The model under review builds one solid part; all positions refer to its coordinate system, in mm. Face numbers are marked on the shaded views. Give positions to 0.01 mm unless a question says otherwise; leave off trailing zeros. Loops run counter-clockwise (first coordinate to the right, second up) from the corner with the lowest first, then second, coordinate; pieces in that order, holes last. Notation, with made-up numbers: M 18.25,62.5 L 67.25,62.5 A23 ccw 67.25,77.5 Z; hole C 76.5,12.5 d11. An arc over 180 degrees is marked long. Write item = value, one per line. Start each with the question number.
1. We need section D-D on x = -3.25. Give the boundary of the cut face in (y, z), then the cut area to 3 significant figures.
2. Draft analysis for pull direction Y (two halves, no side actions). For the marked faces 1, 2 and 3, state which applies: pulls with the +Y half, pulls with the -Y half, needs draft (parallel to the pull), parting line crosses it, or undercut.
3. Wall thickness on line 1 along Y through (x, z) = (0, 7.5); line 2 along Y through (x, z) = (-2.5, 4.25); line 3 along X through (y, z) = (0, 5.25): over which ranges is each line inside the solid? List them lowest first. Write a range as from..to.
4. For pin 1 (4 mm diameter, centred on y = -1.5, z = 6, fed in from +X); pin 2 (1.5 mm diameter, centred on y = -1, z = 5.5, fed in from +X), all flat-tipped, find the tip position at first contact; note any pin that passes through.
5. We need section A-A on x = 0. Give the boundary of the cut face in (y, z).
6. We need section B-B on z = 2. Give the boundary of the cut face in (x, y), then the cut area to 3 significant figures.
7. We need section C-C on y = 0. Give the boundary of the cut face in (x, z), then the cut area to 3 significant figures.
from build123d import *

# Parameters (mm, degrees)
SKETCH1_R           = 4.75
SKETCH1_R_2         = 4
BOSS_EXTRUDE1_DEPTH = 10
CUT_EXTRUDE2_DEPTH  = 10
SKETCH4_W           = 8.174166442
SKETCH4_H           = 1.582309943
BOSS_EXTRUDE2_DEPTH = 0.5


with BuildPart() as part:
    # Sketch1 → Boss-Extrude1 (new body)
    with BuildSketch(Plane.XY):
        Circle(SKETCH1_R)
        Circle(SKETCH1_R_2, mode=Mode.SUBTRACT)
    extrude(amount=BOSS_EXTRUDE1_DEPTH)

    # Sketch3 → Cut-Extrude2 (cut)
    with BuildSketch(Plane.XY.offset(10)):
        with BuildLine():
            ThreePointArc((1.66450103, 3.637229209), (3.365858295, 2.161249162), (4, 0))
            Line((4, 0), (4.75, 0))
            ThreePointArc((4.75, 0), (4.749994219, 0.007410728), (4.749976876, 0.014821438))
            ThreePointArc((4.749976876, 0.014821438), (3.992947753, 2.572716122), (1.976594973, 4.319209686))
            Line((1.976594973, 4.319209686), (1.66450103, 3.637229209))
        make_face()
        with BuildLine():
            Line((4.75, 0), (4, 0))
            ThreePointArc((4, 0), (3.365858295, -2.161249162), (1.66450103, -3.637229209))
            Line((1.66450103, -3.637229209), (1.976594973, -4.319209686))
            ThreePointArc((1.976594973, -4.319209686), (3.996956725, -2.56648338), (4.75, 0))
        make_face()
    extrude(amount=-CUT_EXTRUDE2_DEPTH, mode=Mode.SUBTRACT)

    # Sketch4 → Boss-Extrude2 (add)
    with BuildSketch(Plane(origin=(-4.5, 0, 0), x_dir=(0, 0, -1), z_dir=(1, 0, 0))):
        with Locations((-5.116351143, 0.000178202)):
            Rectangle(SKETCH4_W, SKETCH4_H)
    extrude(amount=-BOSS_EXTRUDE2_DEPTH)


solid = part.part
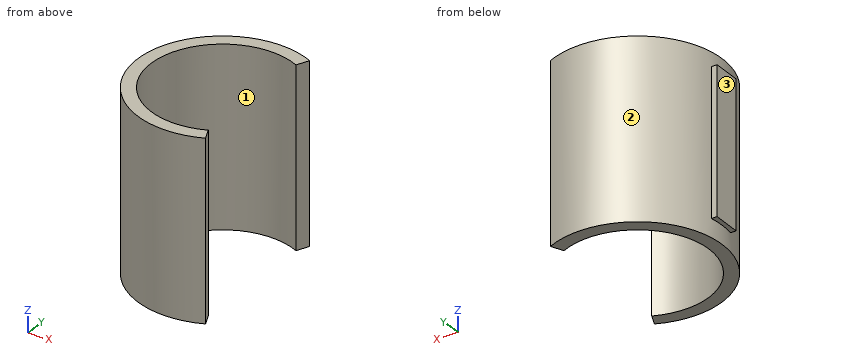
Final values:
q1.outline = M -3.46,0 L -2.33,0 L -2.33,10 L -3.46,10 Z; M 2.33,0 L 3.46,0 L 3.46,10 L 2.33,10 Z
q1.area = 22.6 mm²
q2.face_1 = undercut
q2.face_2 = parting line crosses it
q2.face_3 = needs draft
q3.line_1 = -4.75..-4, 4..4.75
q3.line_2 = -4.04..-3.12, 3.12..4.04
q3.line_3 = -5..-4
q4.pin_1 = -1.94
q4.pin_2 = -3.6
q5.outline = M -4.75,0 L -4,0 L -4,10 L -4.75,10 Z; M 4,0 L 4.75,0 L 4.75,10 L 4,10 Z
q6.outline = M -5,-0.79 L -4.68,-0.79 A4.75 ccw 1.98,-4.32 L 1.66,-3.64 A4 cw long 1.66,3.64 L 1.98,4.32 A4.75 ccw -4.68,0.79 L -5,0.79 Z
q6.area = 13.6 mm²
q7.outline = M -5,1.03 L -4.75,1.03 L -4.75,0 L -4,0 L -4,10 L -4.75,10 L -4.75,9.2 L -5,9.2 Z
q7.area = 9.54 mm²
